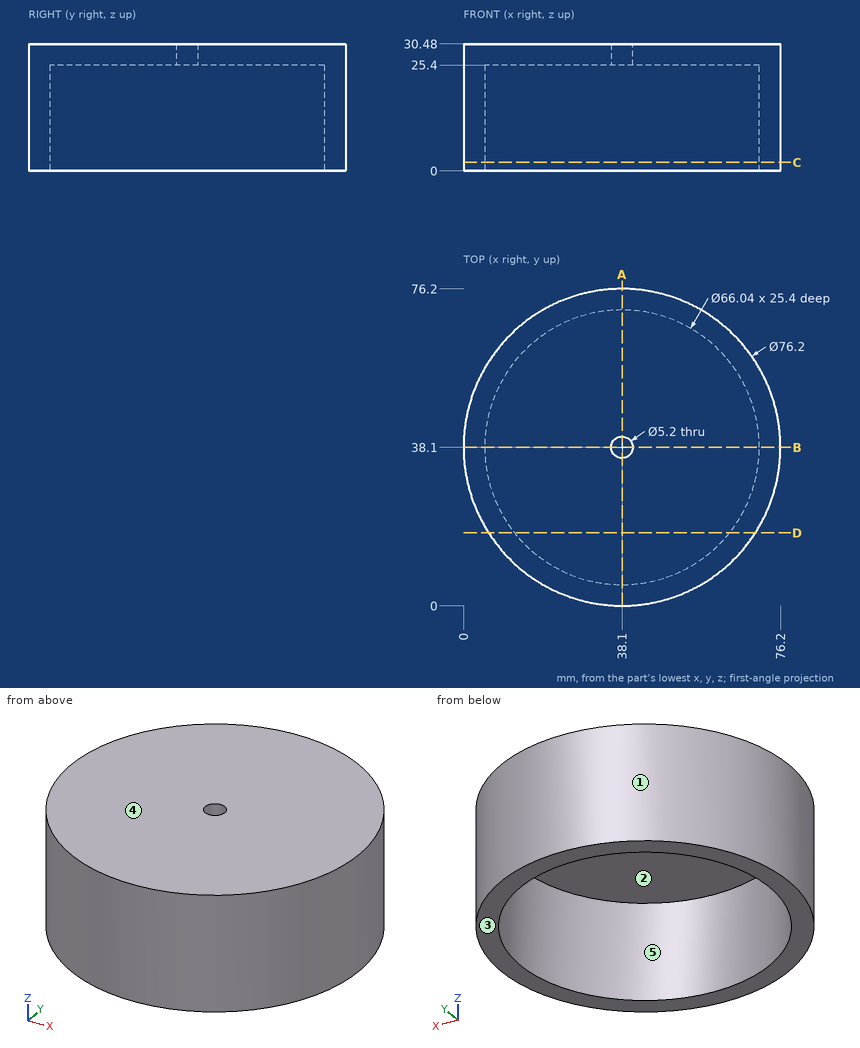
Answer from the drawing. Dimensions are ordinates in mm from the lowest x, y and z of the part. A direction names the side the tool comes from. Round coordinates to 2 decimals unless told otherwise and drop trailing zeros. Loops run counter-clockwise (first coordinate to the right, second up) from the corner with the lowest first, then second, coordinate; pieces in that order, holes last.
Q1. Each of these flat-tipped pins is pushed along its axis until it touches: pin 1 (1 mm diameter, centred on y = 44, z = 8, fed in from -X); pin 2 (1 mm diameter, centred on x = 44, z = 19.5, fed in from +Y); pin 3 (5 mm diameter, centred on y = 27.5, z = 21, fed in from +X); pin 4 (4 mm diameter, centred on x = 38.1, y = 38.1, fed in from +Z). Where does it stop, or does it pass through?
Q2. Which of the six approach directions +Z, -Z, +X, -X, +Y, -Y give full straight-line access (tool end or side, diameter ignored) to the marked faces 4 and 5?
Q3. Consider probe 1 along Y at (x, z) = (38, 15); probe 2 along Y at (x, z) = (38.1, 28.8). Determine where each line is inside the solid, lowest interval first.
Q4. Determine the mould class of the marked faces 1, 2 and 3 for opening direction Y: released by +Y, released by -Y, zero draft, split by the parting line, or undercut.
Q5. Section A-A on x = 38.1 is taken. Write down the section's boundary in (y, z).
Q6. Section C-C on z = 2 is taken. Write down the section's boundary in (x, y).
Q7. Section D-D on y = 17.5 is taken. Write down the section's boundary in (x, z), and give its area (3 significant figures).
Output:
1. pin 1: stops at x = 0.38
1. pin 2: stops at y = 75.82
1. pin 3: stops at x = 75.33
1. pin 4: passes through
2. face 4: +Z, +X, -X, +Y, -Y
2. face 5: -Z
3. probe 1: y = 0 to 5.08, 71.12 to 76.2
3. probe 2: y = 0 to 35.5, 40.7 to 76.2
4. face 1: split by the parting line
4. face 2: undercut
4. face 3: zero draft
5. outline: (0, 0) - (5.08, 0) - (5.08, 25.4) - (35.5, 25.4) - (35.5, 30.48) - (0, 30.48) - close; (40.7, 25.4) - (71.12, 25.4) - (71.12, 0) - (76.2, 0) - (76.2, 30.48) - (40.7, 30.48) - close
6. outline: circle Ø76.2 at (38.1, 38.1); hole circle Ø66.04 at (38.1, 38.1)
7. outline: (6.05, 0) - (12.29, 0) - (12.29, 25.4) - (63.91, 25.4) - (63.91, 0) - (70.15, 0) - (70.15, 30.48) - (6.05, 30.48) - close
7. area: 643 mm2
